CAD build for the part. Positions are in the model's coordinates, mm. A direction names the side the tool comes from. Give positions to 0.01 mm unless a question says otherwise; leave off trailing zeros. Loops run counter-clockwise (first coordinate to the right, second up) from the corner with the lowest first, then second, coordinate; pieces in that order, holes last.
Item 1: Saw through at C-C on x = -3.75. Give the cut face in (y, z), plus the area to 3 significant figures.
Item 2: Probe probe 1 along X at (y, z) = (-3, 5); probe 2 along Z at (x, y) = (6.75, -1); probe 3 along Y at (x, z) = (2.75, -1.25). List the from-to ranges inside material, lowest first.
Item 3: Which spindle directions (+Z, -Z, +X, -X, +Y, -Y) get a long thin tool onto all of the face, cutting with end or side? Do faces 1 (the cylindrical face through (0.09, -1.08, -4.88)), 2 (the flat face through (7.35, -1.2, -1.2)). Say none if no direction does.
Item 4: Saw through at A-A on z = 0. Give the cut face in (x, y), plus the area to 3 significant figures.
Item 5: Drop flat-ended pins along their axis: P1, Ø2, axis at x = 5, z = 4, coming from the -Y side; P2, Ø4, axis at x = 2.5, y = -1, coming from the +Z side. Give the stop position or say it passes through.
Item 6: Mould opens along X. For faces 3 (the flat face through (-7.35, -1.2, 1.2)), 4 (the flat face through (6.35, 4, 4)), 5 (the cylindrical face through (7, 0, 6)) say: released by +X, released by -X, zero draft, split by the parting line, or undercut.
Item 7: Saw through at D-D on y = 3.25. Give the cut face in (x, z).
Autodesk Inventor part; units mm, degrees
ref_plane "YZ Plane" through (0, 0, 0) normal (1, 0, 0) x (0, 1, 0)
ref_plane "XZ Plane" through (0, 0, 0) normal (0, 1, 0) x (-1, 0, 0)
ref_plane "XY Plane" through (0, 0, 0) normal (0, 0, 1) x (1, 0, 0)
sketch "Sketch1" plane through (0, 0, 0) normal (1, 0, 0) x (0, 1, 0)
  circle A0 centre (0, 0) radius 1.5
  circle A1 centre (0, 0) radius 5
  dimension "d0" = 3
  dimension "d1" = 10
extrude "Extrusion1" add sketch "Sketch1" along normal mid plane 12.7
sketch "Sketch2" plane through (6.35, 0, 0) normal (1, 0, 0) x (0, 0, -1)
  circle A0 centre (0, 0) radius 6
  circle A1 centre (0, 0) radius 1.5
  dimension "d4" = 12
  dimension "d5" = 3
extrude "Extrusion2" add sketch "Sketch2" along normal blind 1
mirror "Mirror1" about plane through (0, 0, 0) normal (1, 0, 0) of "Extrusion2"
properties part number "HubV2"
Results below:
1. outline: circle Ø10 at (0, 0); hole circle Ø3 at (0, 0)
1. area: 71.5 mm2
2. probe 1: x = -7.35 to -6.35, 6.35 to 7.35
2. probe 2: z = -5.92 to -1.12, 1.12 to 5.92
2. probe 3: y = -4.84 to -0.83, 0.83 to 4.84
3. face 1: none
3. face 2: +Z, -Z, +X, +Y, -Y
4. outline: (-7.35, -6) - (-6.35, -6) - (-6.35, -5) - (6.35, -5) - (6.35, -6) - (7.35, -6) - (7.35, -1.5) - (-7.35, -1.5) - close; (-7.35, 1.5) - (7.35, 1.5) - (7.35, 6) - (6.35, 6) - (6.35, 5) - (-6.35, 5) - (-6.35, 6) - (-7.35, 6) - close
4. area: 107 mm2
5. P1: stops at y = -4
5. P2: stops at z = 5
6. face 3: released by -X
6. face 4: undercut
6. face 5: zero draft
7. outline: (-7.35, -5.04) - (-6.35, -5.04) - (-6.35, -3.8) - (6.35, -3.8) - (6.35, -5.04) - (7.35, -5.04) - (7.35, 5.04) - (6.35, 5.04) - (6.35, 3.8) - (-6.35, 3.8) - (-6.35, 5.04) - (-7.35, 5.04) - close
